Geometry: final body of the model. Coordinates: model frame, mm. Face numbers are marked on the shaded views. Coordinates: 2 decimals unless noted, no trailing zeros. Loops run counter-clockwise (first coordinate to the right, second up) from the corner with the lowest first, then second, coordinate; pieces in that order, holes last. Notation, with made-up numbers: (27.25, -24.75) - (52.25, -24.75) arc R18 ccw to (52.25, 1.25) - close; hole circle Ø11 at (31, 16.5). An arc over 180 degrees is marked (long way). Answer in a Markdown table with one row per item.
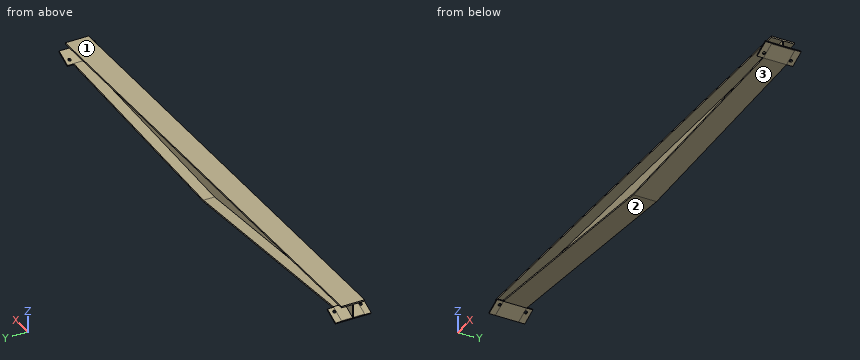
from build123d import *

# Parameters (mm, degrees)
F1_DEPTH = 2.5
F3_DEPTH = 65
F5_W     = 93.2636259532
F5_H     = 200
F5_R     = 8.5
F6_DEPTH = 8
F7_W     = 90
F7_H     = 200
F7_R     = 8.5
F8_DEPTH = 7.33


with BuildPart() as f1:
    # F0 (on Front) → F1 (new body, symmetric)
    with BuildSketch(Plane.XZ):
        Polygon((1400, 140), (0, 140), (-1400, 140), (-1400, 65.3937021232), (-1317.7809088122, 102), (0, 0), (1317.7809088122, 74), (1400, 110.6062978768), align=None)
    extrude(amount=F1_DEPTH, both=True)

    # F2 (on Front) → F3 (join, symmetric)
    with BuildSketch(Plane.XZ):
        Polygon((1317.7809088122, 74), (0, 0), (-1317.7809088122, 102), (-1400, 65.3937021232), (-1400, 57.3697731049), (-1317.7809088122, 93.9760709817), (0, -8.0239290183), (1317.7809088122, 65.9760709817), (1400, 102.5823688585), (1400, 110.6062978768), align=None)
        Polygon((-1400, 140), (0, 140), (1400, 140), (1400, 148), (0, 148), (-1400, 148), align=None)
    extrude(amount=F3_DEPTH, both=True)

    # F5 (on face) → F6 (join)
    with BuildSketch(Plane(origin=(193.4917972476, 0, -434.5896920669), x_dir=(0.9135454576, 0, 0.4067366431), z_dir=(0.4067366431, 0, -0.9135454576))):
        with Locations((1277.3194620245, 0)):
            Rectangle(F5_W, F5_H)
        with Locations((1258.9512750011, -75)):
            Circle(F5_R, mode=Mode.SUBTRACT)
        with Locations((1258.9512750011, 75)):
            Circle(F5_R, mode=Mode.SUBTRACT)
    extrude(amount=-F6_DEPTH)

    # F7 (on face) → F8 (join)
    with BuildSketch(Plane(origin=(-252.9256005596, 0, 568.0801999188), x_dir=(0.9135454576, 0, 0.4067366431), z_dir=(0.4067366431, 0, -0.9135454576))):
        with Locations((-1210.6292517729, 0)):
            Rectangle(F7_W, F7_H)
        with Locations((-1190.6292517729, -73.3960138768)):
            Circle(F7_R, mode=Mode.SUBTRACT)
        with Locations((-1190.6292517729, 73.3960138768)):
            Circle(F7_R, mode=Mode.SUBTRACT)
    extrude(amount=-F8_DEPTH)


solid = f1.part
(1) Ray query, probe 1 along Z at (x, y) = (-851.5, -14); probe 2 along Y at (x, z) = (499.5, 91); probe 3 along Z at (x, y) = (125, -29). Return the intervals inside material, ascending.
Verdict:
| item | result |
|---|---|
| probe 1 | z = 57.88 to 65.91, 140 to 148 |
| probe 2 | y = -2.5 to 2.5 |
| probe 3 | z = -1 to 7.02, 140 to 148 |
(2) Cut plane C-C on x = 1010.5. Output: boundary loops of the cut face in (y, z), then the cut area to 3 significant figures.
Verdict:
| item | result |
|---|---|
| outline | (-65, 48.72) - (65, 48.72) - (65, 56.74) - (2.5, 56.74) - (2.5, 140) - (65, 140) - (65, 148) - (-65, 148) - (-65, 140) - (-2.5, 140) - (-2.5, 56.74) - (-65, 56.74) - close |
| area | 2,500 mm² |
(3) Pull-direction query (X, two-part tool) for the marked faces 1, 2 and 3; classes: pulls with the +X half, pulls with the -X half, needs draft (parallel to the pull), parting line crosses it, or undercut.
Verdict:
| item | result |
|---|---|
| face 1 | needs draft |
| face 2 | undercut |
| face 3 | pulls with the +X half |
(4) Cut plane B-B on x = -1014.5. Output: boundary loops of the cut face in (y, z), then the cut area to 3 significant figures.
Verdict:
| item | result |
|---|---|
| outline | (-65, 70.5) - (65, 70.5) - (65, 78.53) - (2.5, 78.53) - (2.5, 140) - (65, 140) - (65, 148) - (-65, 148) - (-65, 140) - (-2.5, 140) - (-2.5, 78.53) - (-65, 78.53) - close |
| area | 2,390 mm² |
(5) First-contact query: pin 1 Ø6.5 at (x, z) = (-40, 145.5) entering from -Y; pin 2 Ø8 at (y, z) = (-57, 79) entering from +X; pin 3 Ø11 at (y, z) = (-20, 137.5) entering from +X; pin 4 Ø12 at (y, z) = (-36, 100.5) entering from +X. Flat tips, straight axial feed; report the tip coordinate or a pass-through.
Verdict:
| item | result |
|---|---|
| pin 1 | stops at y = -65 |
| pin 2 | stops at x = 1356.02 |
| pin 3 | stops at x = 1400 |
| pin 4 | stops at x = 1402.98 |
